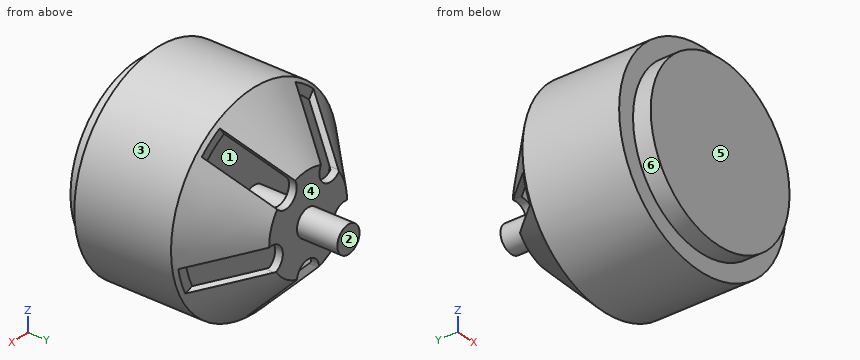
from build123d import *

# Parameters (mm, degrees)
CUT_EXTRUDE1_DEPTH = 15


with BuildPart() as part:
    # Sketch1 → Revolve1 (revolve)
    with BuildSketch(Plane.XY, mode=Mode.PRIVATE) as revolve1_sk:
        Polygon((0, 0), (0, 62), (4, 62), (4, 50), (14.011376117, 50), (30, 34.011376117), (30, 5.271229558), (25, 5.271229558), (25, 0), align=None)
        Polygon((4, 47.694049141), (13.654762603, 47.694049141), (27.337435628, 34.011376117), (4, 34.011376117), align=None, mode=Mode.SUBTRACT)
    revolve(revolve1_sk.sketch.rotate(Axis((0, 0, 0), (0, 1, 0)), 90), axis=Axis((0, 0, 0), (0, 1, 0)))

    # Sketch2 → Cut-Extrude1 (cut)
    with BuildSketch(Plane(origin=(0, 50, 0), x_dir=(1, 0, 0), z_dir=(0, 1, 0))):
        with BuildLine():
            Line((-4, 13.743876759), (-4, 37.242755883))
            Line((-4, 37.242755883), (4, 37.242755883))
            Line((4, 37.242755883), (4, 13.743876759))
            ThreePointArc((4, 13.743876759), (0, 9.743876759), (-4, 13.743876759))
        make_face()
        with BuildLine():
            Line((11.835135573, 8.051317552), (34.18389769, 15.312870551))
            Line((34.18389769, 15.312870551), (36.656033645, 7.70441842))
            Line((36.656033645, 7.70441842), (14.307271528, 0.442865422))
            ThreePointArc((14.307271528, 0.442865422), (9.266977486, 3.01102351), (11.835135573, 8.051317552))
        make_face()
        with BuildLine():
            Line((11.314516046, -8.767888857), (25.126810641, -27.778881418))
            Line((25.126810641, -27.778881418), (18.654674686, -32.481163436))
            Line((18.654674686, -32.481163436), (4.842380091, -13.470170876))
            ThreePointArc((4.842380091, -13.470170876), (5.727307059, -7.882961889), (11.314516046, -8.767888857))
        make_face()
        with BuildLine():
            Line((-4.842380091, -13.470170876), (-18.654674686, -32.481163436))
            Line((-18.654674686, -32.481163436), (-25.126810641, -27.778881418))
            Line((-25.126810641, -27.778881418), (-11.314516046, -8.767888857))
            ThreePointArc((-11.314516046, -8.767888857), (-5.727307059, -7.882961889), (-4.842380091, -13.470170876))
        make_face()
        with BuildLine():
            Line((-14.307271528, 0.442865422), (-36.656033645, 7.70441842))
            Line((-36.656033645, 7.70441842), (-34.18389769, 15.312870551))
            Line((-34.18389769, 15.312870551), (-11.835135573, 8.051317552))
            ThreePointArc((-11.835135573, 8.051317552), (-9.266977486, 3.01102351), (-14.307271528, 0.442865422))
        make_face()
    extrude(amount=-CUT_EXTRUDE1_DEPTH, mode=Mode.SUBTRACT)


solid = part.part
Here's how the part is built. I have some questions about the finished solid (model axes, mm). Face numbers are marked on the shaded views. A direction names the side the tool comes from. Give positions to 0.01 mm unless a question says otherwise; leave off trailing zeros. Order: outer loops, then holes, each group sorted by start corner. A loop starts at its lowest first (then second) coordinate and runs counter-clockwise, first axis right, second up. Notation, with made-up numbers: (67.25, -10.75) -> (126.25, -10.75) arc R12 cw to (126.25, -0.75) -> close; hole circle Ø1 at (29, 45). An arc over 180 degrees is marked (long way). Use a Markdown table: item, result. Add a question column.
Item 1: For the marked faces 4, 5 and 6, which set-ups out of +Z, -Z, +X, -X, +Y, -Y let a thin tool reach every point of the face, with its end or its side?
Item 2: Imagine slicing it at A-A on y = 40.5. Please give me the cut outline in (x, z).
Item 3: Imagine slicing it at B-B on x = 0. Please give me the cut outline in (y, z).
Item 4: Imagine slicing it at D-D on y = 15.5. Please give me the cut outline in (x, z).
Item 5: If we mould it in two halves opening along X, with no side actions, what happens to the marked faces 1, 2 and 3? For each: pulls with the +X half, pulls with the -X half, needs draft (parallel to the pull), parting line crosses it, or undercut.
Item 6: I need wall thicknesses on line 1 (Y direction, x = -6.5, z = -10.5); line 2 (Z direction, x = 1, y = 29); line 3 (Y direction, x = -6, z = -15.5). Which ranges of each line are inside material? Lowest first, please.
Item 7: Imagine slicing it at C-C on y = 56. Please give me the cut outline in (x, z), plus the area to 3 significant figures.
Item 8: Will these pins go through, and if not, where does the flat tip stop? pin 1 (1.5 mm diameter, centred on x = -25.5, z = -9, fed in from +Y); pin 2 (2 mm diameter, centred on x = -23, y = 27, fed in from +Z); pin 3 (4 mm diameter, centred on y = 32.5, z = 22, fed in from -X).
Data:
| question | item | result |
|---|---|---|
| 1 | face 4 | +Y |
| 1 | face 5 | +Z, -Z, +X, -X, -Y |
| 1 | face 6 | -Y |
| 2 | outline | (-23.27, -3.36) -> (-20.7, -2.52) arc R20.85 cw to (-15.26, 14.2) -> (-16.85, 16.39) arc R23.51 ccw to start; (-20.8, -10.96) arc R23.51 ccw to (-4, -23.17) -> (-4, -20.46) arc R20.85 cw to (-18.22, -10.13) -> close; (-10.38, 21.09) -> (-8.79, 18.9) arc R20.85 cw to (8.79, 18.9) -> (10.38, 21.09) arc R23.51 ccw to start; circle Ø8 at (0, 0); (4, -23.17) arc R23.51 ccw to (20.8, -10.96) -> (18.22, -10.13) arc R20.85 cw to (4, -20.46) -> close; (15.26, 14.2) arc R20.85 cw to (20.7, -2.52) -> (23.27, -3.36) arc R23.51 ccw to (16.85, 16.39) -> close |
| 3 | outline | (0, -25) -> (5.27, -25) -> (5.27, -30) -> (34.01, -30) -> (35, -29.01) -> (35, -26.35) -> (34.01, -27.34) -> (34.01, -4) -> (47.69, -4) -> (47.69, -9.74) -> (50, -9.74) -> (50, -4) -> (62, -4) -> (62, 4) -> (50, 4) -> (50, 14.01) -> (34.01, 30) -> (5.27, 30) -> (5.27, 25) -> (0, 25) -> close; hole (34.01, 4) -> (47.69, 4) -> (47.69, 13.65) -> (34.01, 27.34) -> close |
| 4 | outline | circle Ø60 at (0, 0) |
| 5 | face 1 | undercut |
| 5 | face 2 | needs draft |
| 5 | face 3 | parting line crosses it |
| 6 | line 1 | y = 0 to 34.01, 47.69 to 50 |
| 6 | line 2 | z = -29.98 to 29.98 |
| 6 | line 3 | y = 0 to 34.01, 44.73 to 47.39 |
| 7 | outline | circle Ø8 at (0, 0) |
| 7 | area | 50.3 mm² |
| 8 | pin 1 | stops at y = 35 |
| 8 | pin 2 | stops at z = 20.4 |
| 8 | pin 3 | stops at x = -22.36 |
